```python
from build123d import *

# Parameters (mm, degrees)
SKETCH2_W           = 50
SKETCH2_H           = 50
BOSS_EXTRUDE1_DEPTH = 5
FILLET1_R           = 10
SKETCH3_R           = 2.5
CUT_EXTRUDE1_DEPTH  = 6


with BuildPart() as part:
    # Sketch2 → Boss-Extrude1 (new body)
    with BuildSketch(Plane.XY):
        Rectangle(SKETCH2_W, SKETCH2_H)
    extrude(amount=BOSS_EXTRUDE1_DEPTH)

    # Fillet1
    fillet1_edges = [part.edges().sort_by_distance(p)[0] for p in [
        (-25, 25, 2.5),
        (25, 25, 2.5),
        (25, -25, 2.5),
        (-25, -25, 2.5),
    ]]
    fillet(fillet1_edges, radius=FILLET1_R)

    # Sketch3 → Cut-Extrude1 (cut, through all)
    with BuildSketch(Plane.XY.offset(5)):
        with Locations((17.5, 17.5)):
            Circle(SKETCH3_R)
        with BuildLine():
            Line((-5, 0), (-5, -15))
            Line((-5, -15), (-15, -5))
            Line((-15, -5), (-15, 5))
            Line((-15, 5), (-5, 15))
            Line((-5, 15), (-5, 22))
            Line((-5, 22), (5, 22))
            Line((5, 22), (5, 15))
            Line((5, 15), (15, 5))
            Line((15, 5), (15, -5))
            Line((15, -5), (5, -15))
            Line((5, -15), (5, 0))
            ThreePointArc((5, 0), (0, 5), (-5, 0))
        make_face()
    extrude(amount=-CUT_EXTRUDE1_DEPTH, mode=Mode.SUBTRACT)


solid = part.part
```
Read the model definition and answer for the solid it produces. Units are mm, in the model's axes. A direction names the side the tool comes from. Round coordinates to 2 decimals unless told otherwise and drop trailing zeros. Write each loop counter-clockwise with the first axis right and the second up, starting at its lowest first coordinate (ties: lowest second). Pieces come first, ordered by that corner, then holes. Notation, with made-up numbers: (-34, 0.5) -> (-25, 0.5) arc R25 ccw to (-25, 39.5) -> close; hole circle Ø2 at (73, -39). An arc over 180 degrees is marked (long way). Answer in a Markdown table with one row per item. Add a question column.
1) Consider line 1 (X direction, y = -4.5, z = 1.95); line 2 (X direction, y = 18.5, z = 3.2); line 3 (Y direction, x = -7, z = 3.15). Determine where each line is inside the solid, lowest interval first.
2) Which of the six approach directions +Z, -Z, +X, -X, +Y, -Y give full straight-line access (tool end or side, diameter ignored) to faces 1 (the face through (25, 0, 2)), 2 (the face through (10, -10, 3))?
3) Find section C-C, the plane y = -2. Determine the outline of the cut face in (x, z).
4) Determine the mould class of faces 3 (the face through (0, 25, 2)), 4 (the face through (21.99, -22.15, 2.54)), 5 (the face through (0, 5, 3)), 6 (the face through (0, 0, 5)) for opening direction Y: pulls with the +Y half, pulls with the -Y half, needs draft (parallel to the pull), parting line crosses it, or undercut.
5) Given P1, Ø1.5, axis at y = 19, z = 1.5, coming from the +X side, flat-ended and moving along its own axis, determine where the tip first touches the part or whether it passes through.
6) Find section D-D, the plane z = 1.9. Determine the outline of the cut face in (x, y), and give its area (3 significant figures).
7) Find section A-A, the plane x = 0. Determine the outline of the cut face in (y, z), and give its area (3 significant figures).
8) Find section B-B, the plane y = 8. Determine the outline of the cut face in (x, z).
Findings below:
| question | item | result |
|---|---|---|
| 1 | line 1 | -25 to -15, -5 to 5, 15 to 25 |
| 1 | line 2 | -24.37 to -5, 5 to 15.21, 19.79 to 24.37 |
| 1 | line 3 | -25 to -13, 13 to 25 |
| 2 | face 1 | +Z, -Z, +X, +Y, -Y |
| 2 | face 2 | +Z, -Z |
| 3 | outline | (-25, 0) -> (-15, 0) -> (-15, 5) -> (-25, 5) -> close; (-5, 0) -> (5, 0) -> (5, 5) -> (-5, 5) -> close; (15, 0) -> (25, 0) -> (25, 5) -> (15, 5) -> close |
| 4 | face 3 | pulls with the +Y half |
| 4 | face 4 | pulls with the -Y half |
| 4 | face 5 | undercut |
| 4 | face 6 | needs draft |
| 5 | P1 | x = 24.46 |
| 6 | outline | (-25, -15) arc R10 ccw to (-15, -25) -> (15, -25) arc R10 ccw to (25, -15) -> (25, 15) arc R10 ccw to (15, 25) -> (-15, 25) arc R10 ccw to (-25, 15) -> close; hole (-15, -5) -> (-5, -15) -> (-5, 0) arc R5 cw to (5, 0) -> (5, -15) -> (15, -5) -> (15, 5) -> (5, 15) -> (5, 22) -> (-5, 22) -> (-5, 15) -> (-15, 5) -> close; hole circle Ø5 at (17.5, 17.5) |
| 6 | area | 1,810 mm² |
| 7 | outline | (-25, 0) -> (5, 0) -> (5, 5) -> (-25, 5) -> close; (22, 0) -> (25, 0) -> (25, 5) -> (22, 5) -> close |
| 7 | area | 165 mm² |
| 8 | outline | (-25, 0) -> (-12, 0) -> (-12, 5) -> (-25, 5) -> close; (12, 0) -> (25, 0) -> (25, 5) -> (12, 5) -> close |
